Input: part model. Units: mm. Frame: model coordinates. Face numbers are marked on the shaded views. A direction names the side the tool comes from. Round coordinates to 2 decimals unless told otherwise and drop trailing zeros. Order: outer loops, then holes, each group sorted by start corner. A loop starts at its lowest first (then second) coordinate and runs counter-clockwise, first axis right, second up. Notation, with made-up numbers: (-16.75, 31) -> (40.25, 31) arc R30 cw to (40.25, 60) -> close; hole circle Ø10 at (-24, 53). An arc over 180 degrees is marked (long way). Use a Markdown table: item, result.
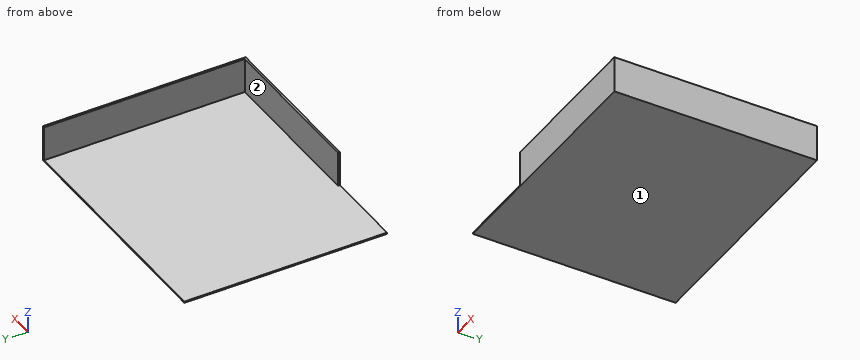
from build123d import *

# Parameters (mm, degrees)
F0_W     = 457.2
F0_H     = 381
F1_DEPTH = 2.54
F2_W     = 304.8
F2_H     = 3.81
F3_DEPTH = 68.58
F4_W     = 3.81
F4_H     = 377.19
F5_DEPTH = 66.04


with BuildPart() as f1:
    # F0 (on Top) → F1 (new body)
    with BuildSketch(Plane.XY):
        with Locations((228.6, 190.5)):
            Rectangle(F0_W, F0_H)
    extrude(amount=F1_DEPTH)

    # F2 (on Top) → F3 (join)
    with BuildSketch(Plane.XY):
        with Locations((304.8, 1.905)):
            Rectangle(F2_W, F2_H)
    extrude(amount=F3_DEPTH)

    # F4 (on face) → F5 (join)
    with BuildSketch(Plane.XY.offset(2.54)):
        with Locations((455.295, 192.405)):
            Rectangle(F4_W, F4_H)
    extrude(amount=F5_DEPTH)


solid = f1.part
1) Set-up query: the marked faces 1 and 2. Return all of +Z, -Z, +X, -X, +Y, -Y with unobstructed straight access to the full face (end or side cutting, diameter ignored); none if empty.
Answer key:
| item | result |
|---|---|
| face 1 | -Z, +X, -X, +Y, -Y |
| face 2 | +Z, -X, +Y |
2) Contact query for flat-ended pins moving along their axis: P1, Ø1.1, axis at y = 2.5, z = 49, coming from the -X side; P2, Ø8, axis at x = 281.5, z = 9, coming from the +Y side. Output: stop coordinate, or through.
Answer key:
| item | result |
|---|---|
| P1 | stops at x = 152.4 |
| P2 | stops at y = 3.81 |
3) Cut plane A-A on x = 196. Return loops of the section in (y, z).
Answer key:
| item | result |
|---|---|
| outline | (0, 0) -> (381, 0) -> (381, 2.54) -> (3.81, 2.54) -> (3.81, 68.58) -> (0, 68.58) -> close |
4) Cut plane C-C on x = 48.5. Return loops of the section in (y, z), and give its area (3 significant figures).
Answer key:
| item | result |
|---|---|
| outline | (0, 0) -> (381, 0) -> (381, 2.54) -> (0, 2.54) -> close |
| area | 968 mm^2 |
5) Ray query, probe 1 along Y at (x, z) = (323.5, 5); probe 2 along Z at (x, y) = (422.5, 20.5); probe 3 along X at (y, z) = (113, 14.5). Return the intervals inside material, ascending.
Answer key:
| item | result |
|---|---|
| probe 1 | y = 0 to 3.81 |
| probe 2 | z = 0 to 2.54 |
| probe 3 | x = 453.39 to 457.2 |
6) Cut plane B-B on y = 171.5. Return loops of the section in (x, z).
Answer key:
| item | result |
|---|---|
| outline | (0, 0) -> (457.2, 0) -> (457.2, 68.58) -> (453.39, 68.58) -> (453.39, 2.54) -> (0, 2.54) -> close |
